The listing builds one solid part. Answer for the finished solid, in the listing's coordinates (mm). A direction names the side the tool comes from. Round coordinates to 2 decimals unless told otherwise and drop trailing zeros. Order: outer loops, then holes, each group sorted by start corner. A loop starts at its lowest first (then second) coordinate and runs counter-clockwise, first axis right, second up. Notation, with made-up numbers: M 32.25,-29.5 L 64.25,-29.5 A19 ccw 64.25,-9.5 Z; hole C 24,-37.5 d7. An arc over 180 degrees is marked long. Write item = value, one per line. Start each with the question number.
(1) Which of the six approach directions +Z, -Z, +X, -X, +Y, -Y give full straight-line access (tool end or side, diameter ignored) to faces 1 (the face through (0.69, -1.44, -5.65)), 2 (the face through (0, -2.2, -4.35)), 3 (the face through (-1.25, 0, -5))?
(2) Straight lines are drawn through the part: probe 1 along Z at (x, y) = (-0.25, 3.25); probe 2 along Z at (x, y) = (0.5, -1) (3 decimals); probe 3 along Y at (x, z) = (-0.5, 3). For each, find the intervals that lie inside material, in ascending order. Write a range as from..to.
(3) A cutting plane is placed at B-B, the plane z = 4. Determine the outline of the cut face in (x, y).
(4) For a pull along Y with two mould halves and no side action, classify faces 4 (the face through (0, 0, 5.65)), 5 (the face through (0.616, -1.088, -5.061)), 6 (the face through (3.233, -1.341, -5.007)) as released by +Y, released by -Y, zero draft, split by the parting line, or undercut.
(5) Each of these flat-tipped pins is pushed along its axis until it touches: pin 1 (1 mm diameter, centred on x = -2, z = -4, fed in from -Y); pin 2 (4 mm diameter, centred on x = 1.5, z = 3.5, fed in from +Y); pin 3 (0.8 mm diameter, centred on x = -0.5, y = -0.5, fed in from -Z) (3 decimals); pin 4 (4 mm diameter, centred on x = 0, z = -3, fed in from +Y). Where does it stop, or does it pass through?
from build123d import *

# Parameters (mm, degrees)
EXTRUDE1_START     = -4.35
SKETCH1_R          = 2
EXTRUDE1_DEPTH     = 10
EXTRUDE2_START     = -5.65
SKETCH6_R          = 3.5
EXTRUDE2_DEPTH     = 1.3
CUT_EXTRUDE1_DEPTH = 0.975
SKETCH8_R          = 1.443375673
CUT_EXTRUDE2_DEPTH = 0.975
CUT_EXTRUDE2_TAPER = 45
CHAMFER1_SIZE      = 0.1625
CHAMFER2_SIZE      = 0.525


with BuildPart() as part:
    # Sketch1 → Extrude1 (new body)
    with BuildSketch(Plane.XY.offset(EXTRUDE1_START)):
        Circle(SKETCH1_R)
    extrude(amount=EXTRUDE1_DEPTH)

    # Sketch6 → Extrude2 (add)
    with BuildSketch(Plane.XY.offset(EXTRUDE2_START)):
        Circle(SKETCH6_R)
    extrude(amount=EXTRUDE2_DEPTH)

    # Sketch7 → Cut-Extrude1 (cut)
    with BuildSketch(Plane.XY.offset(-5.65)):
        Polygon((0, 1.443375673), (-1.25, 0.721687836), (-1.25, -0.721687836), (0, -1.443375673), (1.25, -0.721687836), (1.25, 0.721687836), align=None)
    extrude(amount=CUT_EXTRUDE1_DEPTH, mode=Mode.SUBTRACT)

    # Sketch8 → Cut-Extrude2 (cut)
    with BuildSketch(Plane.XY.offset(-5.65)):
        Circle(SKETCH8_R)
    extrude(amount=CUT_EXTRUDE2_DEPTH, taper=CUT_EXTRUDE2_TAPER, mode=Mode.SUBTRACT)

    # Chamfer1
    chamfer1_edges = [part.edges().sort_by_distance(p)[0] for p in [
        (-3.5, 0, -4.35),
        (-3.5, 0, -5.65),
    ]]
    chamfer(chamfer1_edges, length=CHAMFER1_SIZE)

    # Chamfer2
    chamfer2_edges = [part.edges().sort_by_distance(p)[0] for p in [
        (-2, 0, 5.65),
    ]]
    chamfer(chamfer2_edges, length=CHAMFER2_SIZE)


solid = part.part
Reported:
q1.face_1 = -Z, +X, -X, +Y, -Y
q1.face_2 = +Z
q1.face_3 = -Z
q2.probe_1 = -5.65..-4.35
q2.probe_2 = -4.675..5.65
q2.probe_3 = -1.94..1.94
q3.outline = C 0,0 d4
q4.face_4 = zero draft
q4.face_5 = undercut
q4.face_6 = split by the parting line
q5.pin_1 = -2.94
q5.pin_2 = 2
q5.pin_3 = -4.675
q5.pin_4 = 3.5
